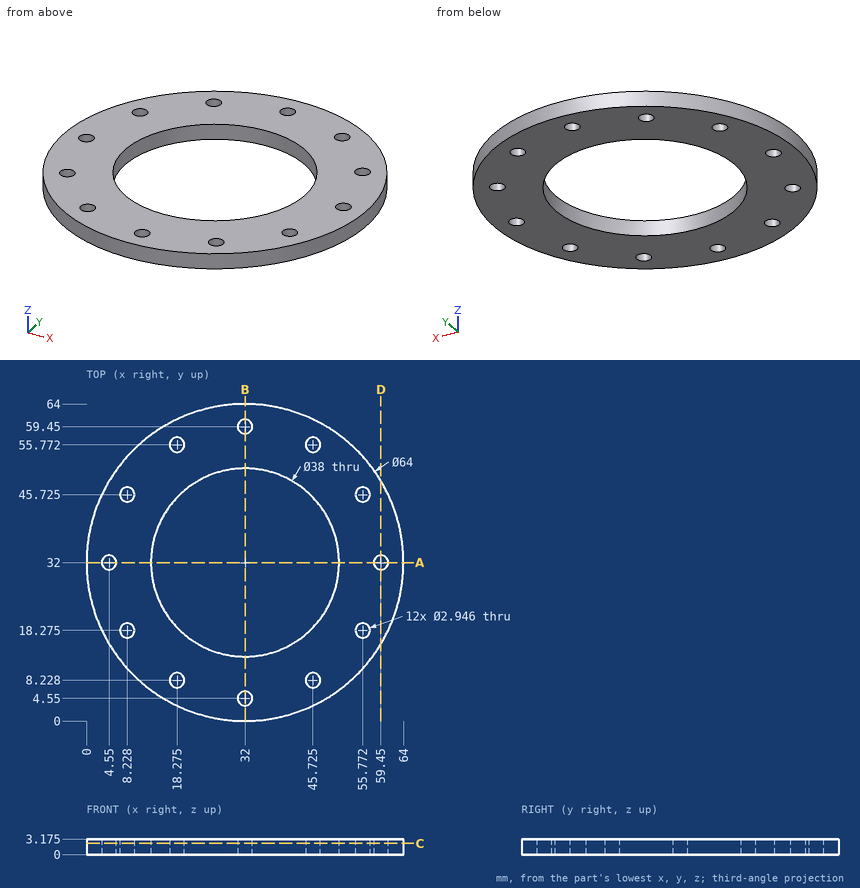
Could you check a few things on this drawing? It's one solid part, dimensions in mm from its lowest x, y, z. Coordinates: 2 decimals unless noted, no trailing zeros. Write each loop counter-clockwise with the first axis right and the second up, starting at its lowest first coordinate (ties: lowest second). Pieces come first, ordered by that corner, then holes. Notation, with made-up numbers: (18.5, 35) - (26.5, 35) arc R18 cw to (26.5, 46) - close; hole circle Ø4 at (43.5, 85.25). An arc over 180 degrees is marked (long way). Use one line per item in the form item = value.
1) I'm going to push flat-ended pins straight in: P1, Ø3.5, axis at x = 55.77, y = 45.72, coming from the -Z side; P2, Ø1.8, axis at x = 8.23, y = 45.72, coming from the +Z side; P3, Ø1, axis at x = 45.5, z = 2, coming from the +Y side; P4, Ø1.5, axis at y = 52.5, z = 2, coming from the +X side. Where does each tip first touch, or does it pass through?
Solved:
P1 = 0
P2 = through
P3 = 61.24
P4 = 57.18
2) Suppose I cut it at D-D, the plane x = 59.45. Write out the boundary of the cut face in (y, z) (1 decimal).
Solved:
outline = (15.6, 0) - (30.5, 0) - (30.5, 3.2) - (15.6, 3.2) - close; (33.5, 0) - (48.4, 0) - (48.4, 3.2) - (33.5, 3.2) - close
3) Suppose I cut it at C-C, the plane z = 2.3. Give the number of separate pieces and of enclosed holes in the cut face, plus the area to 3 significant figures.
Solved:
separate_pieces = 1
enclosed_holes = 13
area = 2,000 mm2
4) Suppose I cut it at A-A, the plane y = 32. Write out the boundary of the cut face in (x, z) (1 decimal).
Solved:
outline = (0, 0) - (3.1, 0) - (3.1, 3.2) - (0, 3.2) - close; (6, 0) - (13, 0) - (13, 3.2) - (6, 3.2) - close; (51, 0) - (58, 0) - (58, 3.2) - (51, 3.2) - close; (60.9, 0) - (64, 0) - (64, 3.2) - (60.9, 3.2) - close
5) I need wall thicknesses on line 1 (Y direction, x = 32, z = 2); line 2 (Y direction, x = 55, z = 1.25); line 3 (X direction, y = 46, z = 0.4) (1 decimal). Which ranges of each line are inside material? Lowest first, please.
Solved:
line_1 = 0 to 3.08, 6.02 to 13, 51 to 57.98, 60.92 to 64
line_2 = 9.75 to 17.02, 19.53 to 44.47, 46.98 to 54.25
line_3 = 3.2 to 6.8, 9.7 to 19.2, 44.8 to 54.3, 57.2 to 60.8
